Work out the finished part from the listing and answer in its coordinate system (mm). A direction names the side the tool comes from. Coordinates: 2 decimals unless noted, no trailing zeros. Write each loop counter-clockwise with the first axis right and the second up, starting at its lowest first coordinate (ties: lowest second). Pieces come first, ordered by that corner, then holes. Notation, with made-up numbers: (-31.5, 85) - (-4.5, 85) arc R17 cw to (-4.5, 106) - close; hole circle Ø10 at (67, 39). An arc over 180 degrees is marked (long way). One line per item, written item: value.
Autodesk Inventor part; units mm, degrees
ref_plane "YZ Plane" through (0, 0, 0) normal (1, 0, 0) x (0, 1, 0)
ref_plane "XZ Plane" through (0, 0, 0) normal (0, 1, 0) x (-1, 0, 0)
ref_plane "XY Plane" through (0, 0, 0) normal (0, 0, 1) x (1, 0, 0)
sketch "Sketch1" plane through (0, 0, 0) normal (0, 1, 0) x (-1, 0, 0)
  line L0 (0, 0) -> (220, 0)
  line L1 (220, 0) -> (220, -100)
  line L2 (220, -100) -> (0, -100)
  line L3 (0, -100) -> (0, 0)
  dimension "d0" = 220
  dimension "d1" = 100
extrude "Extrusion1" add sketch "Sketch1" along normal blind 120
sketch "Sketch2" plane through (0, 120, 0) normal (0, 1, 0) x (1, 0, 0)
  line L0 (-210, 5) -> (-10, 5)
  line L1 (-5, 10) -> (-5, 90)
  line L2 (-10, 95) -> (-210, 95)
  line L3 (-215, 90) -> (-215, 10)
  line L4 (-220, 100) -> (-220, 0)
  line L5 (0, 0) -> (0, 100)
  arc A0 (-210, 95) -> (-215, 90) centre (-210, 90) ccw
  arc A1 (-5, 90) -> (-10, 95) centre (-10, 90) ccw
  arc A2 (-10, 5) -> (-5, 10) centre (-10, 10) ccw
  arc A3 (-215, 10) -> (-210, 5) centre (-210, 10) ccw
  point P0 (-215, 5)
  point P1 (-5, 95)
  point P2 (-5, 5)
  point P3 (-215, 95)
  dimension "d4" = 5
  dimension "d5" = 5
  dimension "d6" = 5
  dimension "d7" = 5
  dimension "d8" = 5
extrude "Extrusion2" cut sketch "Sketch2" against normal blind 115
properties part number "balde"
Item 1: Section C-C, the plane z = -84 is taken. Determine the outline of the cut face in (x, y), then the cut area to 3 significant figures.
Evaluation:
outline: (-220, 0) - (0, 0) - (0, 120) - (-5, 120) - (-5, 5) - (-215, 5) - (-215, 120) - (-220, 120) - close
area: 2,250 mm2
Item 2: Section B-B, the plane x = -126 is taken. Determine the outline of the cut face in (y, z).
Evaluation:
outline: (0, -100) - (120, -100) - (120, -95) - (5, -95) - (5, -5) - (120, -5) - (120, 0) - (0, 0) - close
Item 3: Section A-A, the plane y = 18.5 is taken. Determine the outline of the cut face in (x, z), then the cut area to 3 significant figures.
Evaluation:
outline: (-220, -100) - (0, -100) - (0, 0) - (-220, 0) - close; hole (-215, -90) arc R5 ccw to (-210, -95) - (-10, -95) arc R5 ccw to (-5, -90) - (-5, -10) arc R5 ccw to (-10, -5) - (-210, -5) arc R5 ccw to (-215, -10) - close
area: 3,120 mm2
Item 4: Determine the mould class of faces 3 (the face through (-101, 120, -98)), 4 (the face through (-220, 59, -49)), 5 (the face through (-109, 63, -95)) for opening direction X: +X half, -X half, draft (parallel to the pull), parting line (faces both ways), or undercut.
Evaluation:
face 3: draft
face 4: -X half
face 5: undercut
Item 5: Which of the six approach directions +Z, -Z, +X, -X, +Y, -Y give full straight-line access (tool end or side, diameter ignored) to faces 1 (the face through (-108, 0, -49)), 2 (the face through (-5, 63, -49))?
Evaluation:
face 1: +Z, -Z, +X, -X, -Y
face 2: +Y
Item 6: Consider probe 1 along X at (y, z) = (11.5, -17); probe 2 along Z at (x, y) = (-25, 41); probe 3 along Y at (x, z) = (-178, -79). Determine where each line is inside the solid, lowest interval first.
Evaluation:
probe 1: x = -220 to -215, -5 to 0
probe 2: z = -100 to -95, -5 to 0
probe 3: y = 0 to 5
